from build123d import *

# Parameters (mm, degrees)
SKETCH_R           = 50
PAD_DEPTH          = 10
SKETCH001_R        = 5
POCKET_DEPTH       = 5
POLARPATTERN_COUNT = 10


with BuildPart() as part:
    # Sketch → Pad (new body)
    with BuildSketch(Plane.XY):
        Circle(SKETCH_R)
    extrude(amount=PAD_DEPTH)

    # Sketch001 (on Face3 of Pad) → Pocket (cut)
    with BuildSketch(Plane.XY.offset(10)):
        with Locations((0, 40)):
            Circle(SKETCH001_R)
    pocket = extrude(amount=-POCKET_DEPTH, mode=Mode.SUBTRACT)

    # PolarPattern: Pocket ×10 about axis
    polarpattern_axis = Axis((0, 0, 0), (0, 0, 1))
    for i in range(1, POLARPATTERN_COUNT):
        add(pocket.rotate(polarpattern_axis, i * 360 / POLARPATTERN_COUNT), mode=Mode.SUBTRACT)


solid = part.part
The model under review builds one solid part; all positions refer to its coordinate system, in mm. Give positions to 0.01 mm unless a question says otherwise; leave off trailing zeros. Write each loop counter-clockwise with the first axis right and the second up, starting at its lowest first coordinate (ties: lowest second). Pieces come first, ordered by that corner, then holes.
1. Draft analysis for pull direction X (two halves, no side actions). For faces 1 (the flat face through (-1, 1, 10)), 2 (the cylindrical face through (47.69, 15.02, 4.93)), 3 (the cylindrical face through (-41.22, 16.22, 7.54)), state which applies: +X half, -X half, draft (parallel to the pull), parting line (faces both ways), or undercut.
2. For P1, Ø3, axis at x = 39, y = 13.5, coming from the +Z side; P2, Ø8, axis at x = -21.5, y = -34, coming from the +Z side; P3, Ø1.5, axis at x = -3, z = 1.5, coming from the -Y side; P4, Ø2, axis at y = -23, z = 2, coming from the +X side, all flat-tipped, find the tip position at first contact; note any pin that passes through.
3. Wall thickness on L1, parallel to X at y = 8, z = 8; L2, parallel to Y at x = 24, z = 8; L3, parallel to X at y = 16.5, z = 5.25: over which ranges is each line inside the solid? List them lowest first.
4. Add section B-B, the plane z = 6.75. Count the separate pieces of the cut face and the enclosed holes in it, plus the area to 3 significant figures.
5. Add section D-D, the plane x = -30.5. Write out the cut boundary in (y, z), plus the area to 3 significant figures.
6. Add section A-A, the plane x = 0. Write out the cut boundary in (y, z).
7. Add section C-C, the plane y = -40. Write out the cut boundary in (x, z), plus the area to 3 significant figures.
Worked answers:
1. face 1: draft
1. face 2: parting line
1. face 3: undercut
2. P1: stops at z = 5
2. P2: stops at z = 10
2. P3: stops at y = -49.95
2. P4: stops at x = 44.9
3. L1: x = -49.36 to -40.49, -35.6 to 35.6, 40.49 to 49.36
3. L2: y = -43.86 to -37.34, -27.38 to 27.38, 37.34 to 43.86
3. L3: x = -47.2 to -40.85, -35.24 to 35.24, 40.85 to 47.2
4. separate pieces: 1
4. enclosed holes: 10
4. area: 7,070 mm2
5. outline: (-39.62, 0) - (39.62, 0) - (39.62, 10) - (-39.62, 10) - close
5. area: 792 mm2
6. outline: (-50, 0) - (50, 0) - (50, 10) - (45, 10) - (45, 5) - (35, 5) - (35, 10) - (-35, 10) - (-35, 5) - (-45, 5) - (-45, 10) - (-50, 10) - close
7. outline: (-30, 0) - (30, 0) - (30, 10) - (5, 10) - (5, 5) - (-5, 5) - (-5, 10) - (-30, 10) - close
7. area: 550 mm2
